Check sheet for the modelled part. Datum: model origin and axes. Units: mm. Face numbers are marked on the shaded views. A direction names the side the tool comes from. Round coordinates to 2 decimals unless told otherwise and drop trailing zeros. Write each loop counter-clockwise with the first axis right and the second up, starting at its lowest first coordinate (ties: lowest second). Pieces come first, ordered by that corner, then holes. Notation, with made-up numbers: M 73,54 L 112,54 A28 cw 112,78 Z; hole C 43,49.25 d5. An arc over 180 degrees is marked long. One line per item, written item: value.
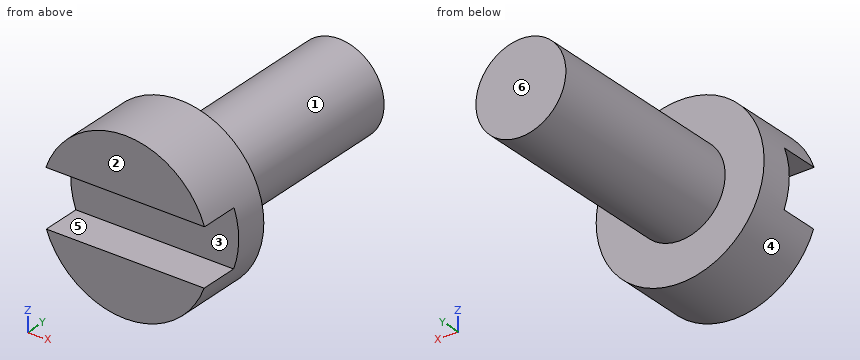
Autodesk Inventor part; units mm, degrees
ref_plane "YZ Plane" through (0, 0, 0) normal (1, 0, 0) x (0, 1, 0)
ref_plane "XZ Plane" through (0, 0, 0) normal (0, 1, 0) x (-1, 0, 0)
ref_plane "XY Plane" through (0, 0, 0) normal (0, 0, 1) x (1, 0, 0)
sketch "Esboço1" plane through (0, 0, 0) normal (0, 1, 0) x (-1, 0, 0)
  circle A0 centre (0, 0) radius 2.8
  dimension "d0" = 5.6
extrude "Extrusão1" add sketch "Esboço1" along normal blind 2.4
sketch "Esboço2" plane through (0, 0, 0) normal (1, 0, 0) x (0, 1, 0)
  line L0 (0, 0.9185) -> (1.2961, 0.9185)
  line L1 (1.2961, 0.9185) -> (1.2961, -0.9611)
  line L2 (1.2961, -0.9611) -> (0, -0.9611)
  line L3 (0, -0.9611) -> (0, 0.9185)
  point P0 (0, 0)
extrude "Extrusão2" cut sketch "Esboço2" along normal through all both and the other way through all
sketch "Esboço3" plane through (0, 2.4, 0) normal (0, 1, 0) x (1, 0, 0)
  circle A0 centre (0, 0) radius 2.8
  circle A1 centre (0, 0) radius 1.5
  dimension "d5" = 3
extrude "Extrusão3" add sketch "Esboço3" along normal blind 7 contours A1
thread "Rosca1"
properties part number "Parafuso-M3-7"
Q1. Sectioned sample at A-A on z = 0. Enter the section's corners in (x, y).
Completed:
outline: M -2.8,1.3 L 2.8,1.3 L 2.8,2.4 L 1.5,2.4 L 1.5,9.4 L -1.5,9.4 L -1.5,2.4 L -2.8,2.4 Z
Q2. Sectioned sample at B-B on x = -1.8. Enter the section's corners in (y, z).
Completed:
outline: M 0,-2.14 L 2.4,-2.14 L 2.4,2.14 L 0,2.14 L 0,0.92 L 1.3,0.92 L 1.3,-0.96 L 0,-0.96 Z
Q3. Depth check by flat-ended pin: P1, Ø1.5, axis at x = 1, z = 0, coming from the -Y side. Enter the tip coordinate at first touch or a pass-through.
Completed:
P1: y = 1.3
Q4. Scan lines: line 1 (Y direction, x = 2.4, z = -0.5); line 2 (Y direction, x = -0.95, z = -0.9); line 3 (Z direction, x = -1.65, y = 1). Record each from-to range of solid material in increasing order. Write a range as [from, to].
Completed:
line 1: [1.3, 2.4]
line 2: [1.3, 9.4]
line 3: [-2.26, -0.96], [0.92, 2.26]
Q5. Access from +Z, -Z, +X, -X, +Y, -Y to the whole of each face (thin tool, end or side, straight path). Record for the marked faces 1, 2 and 3.
Completed:
face 1: +Y
face 2: +Z, -Z, +X, -X, -Y
face 3: +X, -X, -Y
Q6. Sectioned sample at D-D on x = 0. Enter the section's corners in (y, z).
Completed:
outline: M 0,-2.8 L 2.4,-2.8 L 2.4,-1.5 L 9.4,-1.5 L 9.4,1.5 L 2.4,1.5 L 2.4,2.8 L 0,2.8 L 0,0.92 L 1.3,0.92 L 1.3,-0.96 L 0,-0.96 Z
Q7. Draft check along Z on the marked faces 4, 5 and 6. Enter one of: pulls with the +Z half, pulls with the -Z half, needs draft (parallel to the pull), parting line crosses it, or undercut.
Completed:
face 4: parting line crosses it
face 5: undercut
face 6: needs draft
Q8. Sectioned sample at C-C on y = 6.75. Enter the section's corners in (x, z).
Completed:
outline: C 0,0 d3
